```python
from build123d import *

# Parameters (mm, degrees)
SKETCH1_R           = 4.5
BOSS_EXTRUDE1_DEPTH = 50
SKETCH2_R           = 4
CUT_EXTRUDE1_DEPTH  = 50
FILLET2_R           = 1


with BuildPart() as part:
    # Sketch1 → Boss-Extrude1 (new body)
    with BuildSketch(Plane(origin=(0, 0, 0), x_dir=(1, 0, 0), z_dir=(0, 1, 0))):
        with Locations(Location((0, 0, 0), (0, 0, 270))):
            Circle(SKETCH1_R)
    extrude(amount=BOSS_EXTRUDE1_DEPTH)

    # Sketch2 → Cut-Extrude1 (cut)
    with BuildSketch(Plane(origin=(0, 50, 0), x_dir=(1, 0, 0), z_dir=(0, 1, 0))):
        with Locations(Location((0, 0, 0), (0, 0, 270))):
            Circle(SKETCH2_R)
    extrude(amount=-CUT_EXTRUDE1_DEPTH, mode=Mode.SUBTRACT)

    # Fillet2
    # the kernel refuses this fillet: 1 mm, written as the material it takes off along each edge
    with BuildSketch(Plane(origin=(0, 0, 0), x_dir=(0, 0, 1), z_dir=(-1, 0, 0))) as fillet2_piece_1:
        with BuildLine():
            CenterArc((3.5, 0.866025404), FILLET2_R, 300, 60)
            Line((4, 0), (4.01, -0.017320508))
            ThreePointArc((4.01, -0.017320508), (4.25, -0.02), (4.5, -0.02))
            Line((4.5, -0.02), (4.52, 0))
            Line((4.52, 0), (4.52, 0.866025404))
            Line((4.52, 0.866025404), (4.5, 0.866025404))
        make_face()
    revolve(axis=Axis((0, 0, 0), (0, 1, 0)), mode=Mode.SUBTRACT)
    with BuildSketch(Plane(origin=(0, 50, 0), x_dir=(0, 0, 1), z_dir=(-1, 0, 0))) as fillet2_piece_2:
        with BuildLine():
            CenterArc((3.5, -0.866025404), FILLET2_R, 0, 60)
            Line((4, 0), (4.01, 0.017320508))
            ThreePointArc((4.01, 0.017320508), (4.25, 0.02), (4.5, 0.02))
            Line((4.5, 0.02), (4.52, 0))
            Line((4.52, 0), (4.52, -0.866025404))
            Line((4.52, -0.866025404), (4.5, -0.866025404))
        make_face()
    revolve(axis=Axis((0, 50, 0), (0, 1, 0)), mode=Mode.SUBTRACT)


solid = part.part
```
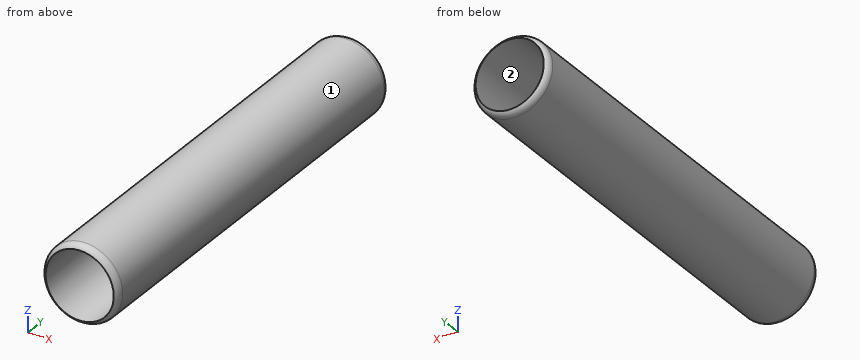
The listing builds one solid part. Answer for the finished solid, in the listing's coordinates (mm). Face numbers are marked on the shaded views. Round coordinates to 2 decimals unless told otherwise and drop trailing zeros. Order: outer loops, then holes, each group sorted by start corner. A loop starts at its lowest first (then second) coordinate and runs counter-clockwise, first axis right, second up. Notation, with made-up numbers: (17, 22) - (31, 22) arc R33 ccw to (31, 58) - close; hole circle Ø2 at (-20.5, 89). An arc over 180 degrees is marked (long way). Put each result on its own line as item: value. Start each with the question number.
(1) Find section C-C (y = 29). Give the vertices of the cut face in (x, z).
(2) Given P1, Ø2, axis at y = 41, z = -3, coming from the +X side; P2, Ø2, axis at y = 28.5, z = -3.5, coming from the +X side, each flat-ended and moving along its own axis, determine where each tip first touches the part or whether it passes through.
(3) Determine the mould class of the marked faces 1 and 2 for opening direction X: released by +X, released by -X, zero draft, split by the parting line, or undercut.
(4) Find section A-A (z = 0). Give the vertices of the cut face in (x, y), plus the area to 3 significant figures.
(5) Find section B-B (x = 0). Give the vertices of the cut face in (y, z), plus the area to 3 significant figures.
(6) Straight lines are drawn through the part: probe 1 along X at (y, z) = (13, 0); probe 2 along X at (y, z) = (35, -3.25); probe 3 along Z at (x, y) = (-3, 29). For each, find the intervals that lie inside material, in ascending order. Write a range as from..to.
Reply:
1. outline: circle Ø9 at (0, 0); hole circle Ø8 at (0, 0)
2. P1: x = 4.03
2. P2: x = 3.74
3. face 1: split by the parting line
3. face 2: undercut
4. outline: (-4.5, 0.87) arc R1 ccw to (-4, 0) - (-4, 50) arc R1 ccw to (-4.5, 49.13) - close; (4, 0) arc R1 ccw to (4.5, 0.87) - (4.5, 49.13) arc R1 ccw to (4, 50) - close
4. area: 49.5 mm^2
5. outline: (0, -4) arc R1 ccw to (0.87, -4.5) - (49.13, -4.5) arc R1 ccw to (50, -4) - close; (0, 4) - (50, 4) arc R1 ccw to (49.13, 4.5) - (0.87, 4.5) arc R1 ccw to start
5. area: 49.5 mm^2
6. probe 1: -4.5..-4, 4..4.5
6. probe 2: -3.11..-2.33, 2.33..3.11
6. probe 3: -3.35..-2.65, 2.65..3.35
